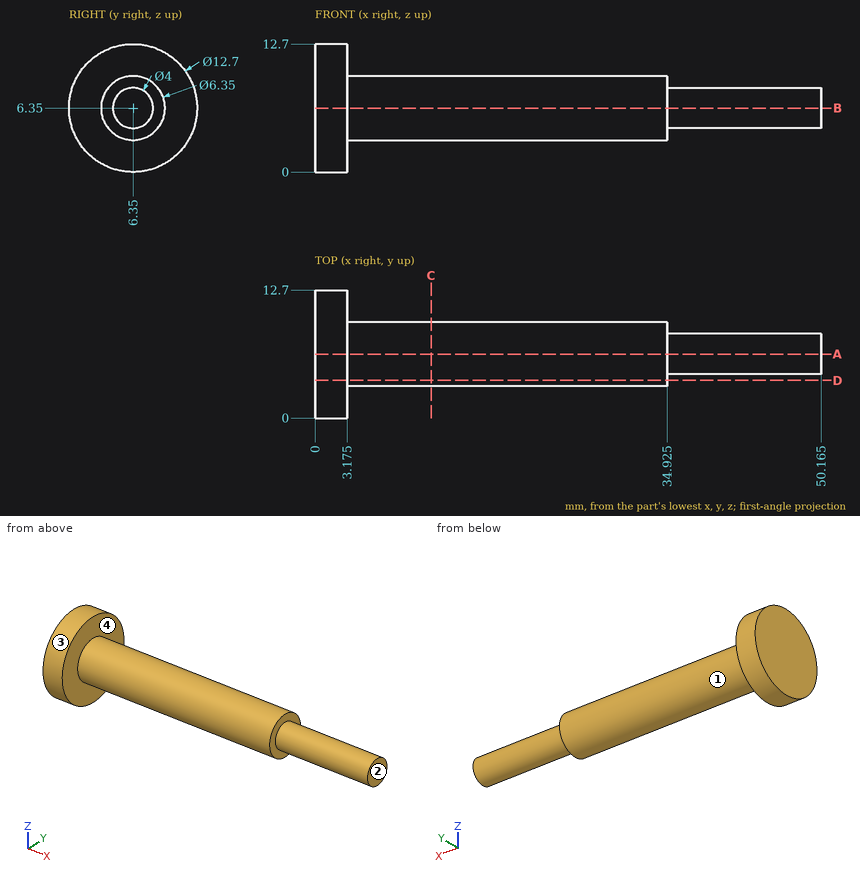
Geometry check sheet. Reference: drawing and pictorial views, mm from the part's lowest x, y, z. A direction names the side the tool comes from. Round coordinates to 2 decimals unless told otherwise and drop trailing zeros. Loops run counter-clockwise (first coordinate to the right, second up) from the corner with the lowest first, then second, coordinate; pieces in that order, holes last. Notation, with made-up numbers: (34.25, 87) - (70.25, 87) arc R19 cw to (70.25, 119) - close; hole circle Ø11 at (10.5, 72.25). An arc over 180 degrees is marked (long way). Use a Markdown table: item, result.
Q1. Go/stop test with flat-tipped pins: P1, Ø6, axis at x = 27, y = 9, coming from the -Z side (3 decimals); P2, Ø1.5, axis at x = 36, y = 5, coming from the -Z side; P3, Ø2, axis at x = 44.5, z = 7.5, coming from the -Y side. Record where each tip stops, or that it passes through.
Solutions:
| item | result |
|---|---|
| P1 | stops at z = 3.175 |
| P2 | stops at z = 4.44 |
| P3 | stops at y = 4.36 |
Q2. Cross-section at C-C on x = 11.5. Record the cut outline in (y, z) (3 decimals), plus the area to 3 significant figures.
Solutions:
| item | result |
|---|---|
| outline | circle Ø6.35 at (6.35, 6.35) |
| area | 31.7 mm2 |
Q3. Cross-section at D-D on y = 3.75. Record the cut outline in (x, z) (3 decimals).
Solutions:
| item | result |
|---|---|
| outline | (0, 0.557) - (3.175, 0.557) - (3.175, 4.528) - (34.925, 4.528) - (34.925, 8.172) - (3.175, 8.172) - (3.175, 12.143) - (0, 12.143) - close |
Q4. Cross-section at A-A on y = 6.35. Record the cut outline in (x, z) (3 decimals).
Solutions:
| item | result |
|---|---|
| outline | (0, 0) - (3.175, 0) - (3.175, 3.175) - (34.925, 3.175) - (34.925, 4.35) - (50.165, 4.35) - (50.165, 8.35) - (34.925, 8.35) - (34.925, 9.525) - (3.175, 9.525) - (3.175, 12.7) - (0, 12.7) - close |
Q5. Material ranges on line 1 (X direction, y = 2, z = 3.5) (3 decimals); line 2 (X direction, y = 7.25, z = 4.5) (3 decimals); line 3 (Z direction, x = 16.5, y = 8.5), recorded low to high.
Solutions:
| item | result |
|---|---|
| line 1 | x = 0 to 3.175 |
| line 2 | x = 0 to 34.925 |
| line 3 | z = 4.01 to 8.69 |
Q6. Draft check along Z on the marked faces 1 and 2. Enter one of: released by +Z, released by -Z, zero draft, split by the parting line, or undercut.
Solutions:
| item | result |
|---|---|
| face 1 | split by the parting line |
| face 2 | zero draft |
Q7. Access from +Z, -Z, +X, -X, +Y, -Y to the whole of each face (thin tool, end or side, straight path). Record for the marked faces 3 and 4.
Solutions:
| item | result |
|---|---|
| face 3 | +X, -X |
| face 4 | +X |
